Work out the finished part from the listing and answer in its coordinate system (mm). A direction names the side the tool comes from. Give positions to 0.01 mm unless a question says otherwise; leave off trailing zeros. Loops run counter-clockwise (first coordinate to the right, second up) from the corner with the lowest first, then second, coordinate; pieces in that order, holes last. Notation, with made-up numbers: M 63.25,-28.75 L 109.25,-28.75 A18 ccw 109.25,-14.75 Z; hole C 47.25,87 d11. An arc over 180 degrees is marked long. Answer in a Markdown table with one row per item. Add a question column.
from build123d import *

# Parameters (mm, degrees)
F0_W     = 5.08
F0_H     = 4.0894
F0_W_2   = 20.32
F0_H_2   = 50.8
F1_DEPTH = 4.0894


with BuildPart() as f1:
    # F0 (on Top) → F1 (new body)
    with BuildSketch(Plane.XY):
        Polygon((21.59, -2.0447), (15.24, -2.0447), (10.16, -2.0447), (-10.16, -2.0447), (-15.24, -2.0447), (-21.59, -2.0447), (-21.59, -8.3947), (-10.16, -8.3947), (10.16, -8.3947), (21.59, -8.3947), align=None)
        with Locations((12.7, 0)):
            Rectangle(F0_W, F0_H)
        with Locations((-12.7, 0)):
            Rectangle(F0_W, F0_H)
        with Locations((0, -33.7947)):
            Rectangle(F0_W_2, F0_H_2)
        Polygon((21.59, -59.1947), (10.16, -59.1947), (-10.16, -59.1947), (-21.59, -59.1947), (-21.59, -65.5447), (-15.24, -65.5447), (-10.16, -65.5447), (10.16, -65.5447), (15.24, -65.5447), (21.59, -65.5447), align=None)
        with Locations((12.7, -67.5894)):
            Rectangle(F0_W, F0_H)
        with Locations((-12.7, -67.5894)):
            Rectangle(F0_W, F0_H)
    extrude(amount=F1_DEPTH)


solid = f1.part
(1) Consider line 1 along X through (y, z) = (-1.5, 0.4); line 2 along Y through (x, z) = (11.5, 0.3); line 3 along Y through (x, z) = (17, 3.6). Determine where each line is inside the solid, lowest interval first. Write a range as from..to.
(2) The mould has two halves that part along X. Classify faces 6 (the face through (16, -59.195, 2)), 7 (the face through (-15.24, 0, 2)), 8 (the face through (-10.16, -68, 2)): pulls with the +X half, pulls with the -X half, needs draft (parallel to the pull), parting line crosses it, or undercut.
(3) Section D-D, the plane y = -30.5 is taken. Determine the outline of the cut face in (x, z).
(4) Section C-C, the plane z = 1.75 is taken. Determine the outline of the cut face in (x, y), and give its area (3 significant figures).
(5) Section B-B, the plane x = 16 is taken. Determine the outline of the cut face in (y, z).
(6) Section A-A, the plane x = -11 is taken. Determine the outline of the cut face in (y, z).
(7) Each of these flat-tipped pins is pushed along its axis until it touches: P1, Ø2, axis at y = -41.5, z = 2.5, coming from the +X side; P2, Ø1.5, axis at x = 4.5, y = -33.5, coming from the -Z side; P3, Ø1.2, axis at x = 4.5, z = 1, coming from the -Y side; P4, Ø1.2, axis at y = -24, z = 2.5, coming from the -X side. Where does it stop, or does it pass through?
(8) Which of the six approach directions +Z, -Z, +X, -X, +Y, -Y give full straight-line access (tool end or side, diameter ignored) to faces 1 (the face through (15.24, 0, 2)), 2 (the face through (15.24, -68, 2)), 3 (the face through (-18, -2.045, 2)), 4 (the face through (-16, -59.195, 2)), 5 (the face through (-15.24, -68, 2))?
Numbers:
| question | item | result |
|---|---|---|
| 1 | line 1 | x = -15.24..-10.16, 10.16..15.24 |
| 1 | line 2 | y = -69.63..-59.19, -8.39..2.04 |
| 1 | line 3 | y = -65.54..-59.19, -8.39..-2.04 |
| 2 | face 6 | needs draft |
| 2 | face 7 | pulls with the -X half |
| 2 | face 8 | undercut |
| 3 | outline | M -10.16,0 L 10.16,0 L 10.16,4.09 L -10.16,4.09 Z |
| 4 | outline | M -21.59,-65.54 L -15.24,-65.54 L -15.24,-69.63 L -10.16,-69.63 L -10.16,-65.54 L 10.16,-65.54 L 10.16,-69.63 L 15.24,-69.63 L 15.24,-65.54 L 21.59,-65.54 L 21.59,-59.19 L 10.16,-59.19 L 10.16,-8.39 L 21.59,-8.39 L 21.59,-2.04 L 15.24,-2.04 L 15.24,2.04 L 10.16,2.04 L 10.16,-2.04 L -10.16,-2.04 L -10.16,2.04 L -15.24,2.04 L -15.24,-2.04 L -21.59,-2.04 L -21.59,-8.39 L -10.16,-8.39 L -10.16,-59.19 L -21.59,-59.19 Z |
| 4 | area | 1,660 mm² |
| 5 | outline | M -65.54,0 L -59.19,0 L -59.19,4.09 L -65.54,4.09 Z; M -8.39,0 L -2.04,0 L -2.04,4.09 L -8.39,4.09 Z |
| 6 | outline | M -69.63,0 L -59.19,0 L -59.19,4.09 L -69.63,4.09 Z; M -8.39,0 L 2.04,0 L 2.04,4.09 L -8.39,4.09 Z |
| 7 | P1 | stops at x = 10.16 |
| 7 | P2 | stops at z = 0 |
| 7 | P3 | stops at y = -65.54 |
| 7 | P4 | stops at x = -10.16 |
| 8 | face 1 | +Z, -Z, +X, +Y |
| 8 | face 2 | +Z, -Z, +X, -Y |
| 8 | face 3 | +Z, -Z, -X, +Y |
| 8 | face 4 | +Z, -Z, -X |
| 8 | face 5 | +Z, -Z, -X, -Y |
